Input: part model. Units: mm. Frame: model coordinates. A direction names the side the tool comes from. Give positions to 0.01 mm unless a question says otherwise; leave off trailing zeros. Loops run counter-clockwise (first coordinate to the right, second up) from the corner with the lowest first, then second, coordinate; pieces in that order, holes last. Notation, with made-up numbers: (16.5, 45.25) -> (71.5, 45.25) arc R8 cw to (71.5, 51.25) -> close; hole circle Ø2 at (35.25, -13). An arc over 180 degrees is marked (long way). Answer as a JSON object with one key per item and string values.
```python
from build123d import *

# Parameters (mm, degrees)
ESQUISSE1_W             = 88
ESQUISSE1_H             = 88
BOSS_EXTRU_1_DEPTH      = 6
ESQUISSE2_R             = 5
ENL_V_MAT_EXTRU_1_DEPTH = 6
ESQUISSE3_W             = 88
ESQUISSE3_H             = 50
BOSS_EXTRU_2_DEPTH      = 6
ESQUISSE4_W             = 50
ESQUISSE4_H             = 94
BOSS_EXTRU_3_DEPTH      = 6
ESQUISSE5_W             = 50
ESQUISSE5_H             = 94
BOSS_EXTRU_4_DEPTH      = 6
ESQUISSE6_W             = 100
ESQUISSE6_H             = 50
BOSS_EXTRU_5_DEPTH      = 6
ESQUISSE7_R             = 1
ENL_V_MAT_EXTRU_2_DEPTH = 100


with BuildPart() as part:
    # Esquisse1 → Boss.-Extru.1 (new body)
    with BuildSketch(Plane.XY):
        Rectangle(ESQUISSE1_W, ESQUISSE1_H)
    extrude(amount=BOSS_EXTRU_1_DEPTH)

    # Esquisse2 → Enlèv. mat.-Extru.1 (cut)
    with BuildSketch(Plane.XY.offset(6)):
        Circle(ESQUISSE2_R)
    extrude(amount=-ENL_V_MAT_EXTRU_1_DEPTH, mode=Mode.SUBTRACT)

    # Esquisse3 → Boss.-Extru.2 (add)
    with BuildSketch(Plane(origin=(0, -44, 0), x_dir=(-1, 0, 0), z_dir=(0, -1, 0))):
        with Locations((0, -25)):
            Rectangle(ESQUISSE3_W, ESQUISSE3_H)
    extrude(amount=BOSS_EXTRU_2_DEPTH)

    # Esquisse4 → Boss.-Extru.3 (add)
    with BuildSketch(Plane.ZY.offset(44)):
        with Locations((25, -3)):
            Rectangle(ESQUISSE4_W, ESQUISSE4_H)
    extrude(amount=BOSS_EXTRU_3_DEPTH)

    # Esquisse5 → Boss.-Extru.4 (add)
    with BuildSketch(Plane(origin=(44, 0, 0), x_dir=(0, 0, -1), z_dir=(1, 0, 0))):
        with Locations((-25, -3)):
            Rectangle(ESQUISSE5_W, ESQUISSE5_H)
    extrude(amount=BOSS_EXTRU_4_DEPTH)

    # Esquisse6 → Boss.-Extru.5 (add)
    with BuildSketch(Plane(origin=(0, 44, 0), x_dir=(1, 0, 0), z_dir=(0, 1, 0))):
        with Locations((0, -25)):
            Rectangle(ESQUISSE6_W, ESQUISSE6_H)
    extrude(amount=BOSS_EXTRU_5_DEPTH)

    # Esquisse7 → Enlèv. mat.-Extru.2 (cut)
    with BuildSketch(Plane(origin=(0, 50, 0), x_dir=(1, 0, 0), z_dir=(0, 1, 0))):
        with Locations(Location((35, -10, 0), (0, 0, 270))):
            Circle(ESQUISSE7_R)
        with Locations(Location((-35, -10, 0), (0, 0, 270))):
            Circle(ESQUISSE7_R)
    extrude(amount=-ENL_V_MAT_EXTRU_2_DEPTH, mode=Mode.SUBTRACT)


solid = part.part
```
Q1. Access query for faces 5 (the flat face through (-45, 0, 50)), 6 (the flat face through (1, -44, 28)). Directions: +Z, -Z, +X, -X, +Y, -Y. A direction counts if a zero-diameter tool reaches every point of the face in a straight line with its end or side. Return the directions, or none.
Evaluation:
{"face 5": "+Z, +X, -X, +Y, -Y", "face 6": "+Z"}
Q2. Section C-C, the plane x = -28. Return the cut outline in (y, z), then the cut area to 3 significant figures.
Evaluation:
{"outline": "(-50, 0) -> (50, 0) -> (50, 50) -> (44, 50) -> (44, 6) -> (-44, 6) -> (-44, 50) -> (-50, 50) -> close", "area": "1,130 mm2"}
Q3. Section B-B, the plane x = 0. Return the cut outline in (y, z), then the cut area to 3 significant figures.
Evaluation:
{"outline": "(-50, 0) -> (-5, 0) -> (-5, 6) -> (-44, 6) -> (-44, 50) -> (-50, 50) -> close; (5, 0) -> (50, 0) -> (50, 50) -> (44, 50) -> (44, 6) -> (5, 6) -> close", "area": "1,070 mm2"}
Q4. Ray query, line 1 along X through (y, z) = (-46, 10); line 2 along Y through (x, z) = (13.5, 18.5). Return the intervals inside material, ascending.
Evaluation:
{"line 1": "x = -50 to -36, -34 to 34, 36 to 50", "line 2": "y = -50 to -44, 44 to 50"}
Q5. Pin query (flat end, axial travel): pin 1 (8 mm diameter, centred on x = 0, y = 0, fed in from +Z); pin 2 (1.5 mm diameter, centred on x = -20.5, y = -32, fed in from +Z). Return the tip coordinate at first contact, or that it passes through.
Evaluation:
{"pin 1": "passes through", "pin 2": "stops at z = 6"}
Q6. Section A-A, the plane z = 40.5. Return the cut outline in (x, y).
Evaluation:
{"outline": "(-50, -50) -> (50, -50) -> (50, 50) -> (-50, 50) -> close; hole (-44, -44) -> (44, -44) -> (44, 44) -> (-44, 44) -> close"}
Q7. Draft query along Y for faces 1 (the flat face through (50, -1, 25)), 2 (the flat face through (-1, -50, 25)), 3 (the flat face through (-44, 1, 28)), 4 (the flat face through (-1, 50, 25)). Return one class per face: +Y half, -Y half, draft (parallel to the pull), parting line (faces both ways), or undercut.
Evaluation:
{"face 1": "draft", "face 2": "-Y half", "face 3": "undercut", "face 4": "+Y half"}
